from build123d import *

# Parameters (mm, degrees)
SKETCH1_R               = 30.1625
SKETCH1_R_2             = 25.4
BOSS_EXTRUDE1_DEPTH     = 812.8
CUT_EXTRUDE2_DEPTH      = 814.918541878
CUT_EXTRUDE2_DEPTH_BACK = 814.918541878
SKETCH4_R               = 2.54
SKETCH4_W               = 15.875
SKETCH4_H               = 6.35


with BuildPart() as part:
    # Sketch1 → Boss-Extrude1 (new body)
    with BuildSketch(Plane(origin=(0, 0, 0), x_dir=(1, 0, 0), z_dir=(0, 1, 0))):
        with Locations(Location((0, 0, 0), (0, 0, 270))):
            Circle(SKETCH1_R)
        with Locations(Location((0, 0, 0), (0, 0, 270))):
            Circle(SKETCH1_R_2, mode=Mode.SUBTRACT)
    extrude(amount=BOSS_EXTRUDE1_DEPTH)

    # Sketch4 → Cut-Extrude2 (cut, two sides: drawn at the far end of the back side and taken through both)
    with BuildSketch(Plane.XY.offset(-CUT_EXTRUDE2_DEPTH_BACK)):
        with Locations((0, 685.8)):
            Circle(SKETCH4_R)
        with Locations((0, 788.9875)):
            Circle(SKETCH4_R)
        with Locations((22.225, 796.925)):
            Rectangle(SKETCH4_W, SKETCH4_H)
    extrude(amount=CUT_EXTRUDE2_DEPTH + CUT_EXTRUDE2_DEPTH_BACK, mode=Mode.SUBTRACT)


solid = part.part
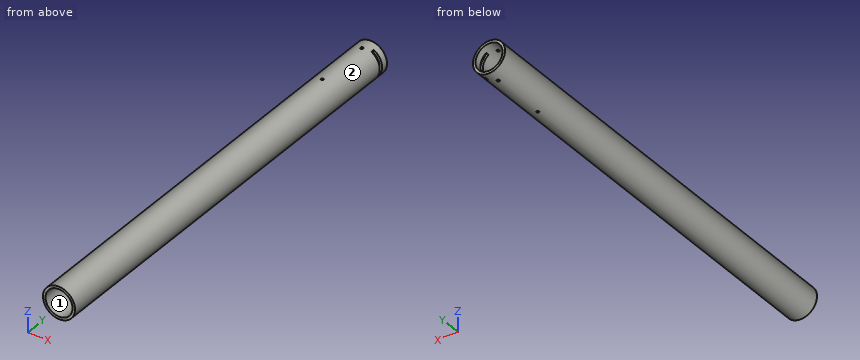
Read the model definition and answer for the solid it produces. Units are mm, in the model's axes. Face numbers are marked on the shaded views. Coordinates: 2 decimals unless noted, no trailing zeros. Order: outer loops, then holes, each group sorted by start corner. A loop starts at its lowest first (then second) coordinate and runs counter-clockwise, first axis right, second up. Notation, with made-up numbers: M 48,32.5 L 92,32.5 A12 cw 92,41.5 Z; hole C 50.25,16 d9. An arc over 180 degrees is marked long. Put each result on its own line as item: value. Start each with the question number.
Item 1: Section A-A, the plane z = 0 is taken. Determine the outline of the cut face in (x, y).
Item 2: The mould has two halves that part along Z. Classify the marked faces 1 and 2: +Z half, -Z half, draft (parallel to the pull), parting line (faces both ways), or undercut.
Item 3: Section B-B, the plane y = 366 is taken. Determine the outline of the cut face in (x, z) (1 decimal), plus the area to 3 significant figures.
Item 4: Section C-C, the plane x = -16.5 is taken. Determine the outline of the cut face in (y, z), plus the area to 3 significant figures.
Item 5: Given pin 1 Ø4.5 at (y, z) = (798.5, -23) entering from +X; pin 2 Ø1.7 at (y, z) = (795.5, 24.5) entering from +X; pin 3 Ø8 at (y, z) = (684, 21.5) entering from -X; pin 4 Ø4 at (x, y) = (0, 788.99) entering from +Z, each flat-ended and moving along its own axis, determine where each tip first touches the part or whether it passes through.
Item 6: Consider probe 1 along Y at (x, z) = (0, 27.55); probe 2 along Z at (x, y) = (3, 333); probe 3 along Z at (x, y) = (0, 458). Determine where each line is inside the solid, lowest interval first. Write a range as [from, to].
Computed:
1. outline: M -30.16,0 L -25.4,0 L -25.4,812.8 L -30.16,812.8 Z; M 25.4,0 L 30.16,0 L 30.16,793.75 L 25.4,793.75 Z; M 25.4,800.1 L 30.16,800.1 L 30.16,812.8 L 25.4,812.8 Z
2. face 1: undercut
2. face 2: parting line
3. outline: C 0,0 d60.3; hole C 0,0 d50.8
3. area: 831 mm2
4. outline: M 0,-25.25 L 812.8,-25.25 L 812.8,-19.31 L 0,-19.31 Z; M 0,19.31 L 812.8,19.31 L 812.8,25.25 L 0,25.25 Z
4. area: 9,650 mm2
5. pin 1: stops at x = 21.24
5. pin 2: stops at x = 14.29
5. pin 3: stops at x = -24.57
5. pin 4: passes through
6. probe 1: y = [0, 683.26], [688.34, 786.45], [791.53, 812.8]
6. probe 2: z = [-30.01, -25.22], [25.22, 30.01]
6. probe 3: z = [-30.16, -25.4], [25.4, 30.16]
